from build123d import *

# Parameters (mm, degrees)
BOSS_EXTRUDE5_DEPTH      = 69.85
BOSS_EXTRUDE5_DEPTH_BACK = 19.05
SKETCH1_R                = 25.4
SKETCH1_R_2              = 2.38125
SKETCH1_R_3              = 15.875
SKETCH2_R                = 190.5
SKETCH2_R_2              = 25.4
BOSS_EXTRUDE7_DEPTH      = 69.85
SKETCH4_R                = 190.5
SKETCH4_R_2              = 25.4
CUT_EXTRUDE2_DEPTH       = 19.05
FILLET1_R                = 25.4


with BuildPart() as part:
    # Sketch1 → Boss-Extrude5 (new, two sides: drawn at the far end of the back side and taken through both)
    with BuildSketch(Plane(origin=(0, 0, 0), x_dir=(1, 0, 0), z_dir=(0, 1, 0)).offset(-BOSS_EXTRUDE5_DEPTH_BACK)):
        with Locations(Location((0, 0, 0), (0, 0, 270))):
            Circle(SKETCH1_R)
        with Locations(Location((-8.954275666, 18.593745011, 0), (0, 0, 270))):
            Circle(SKETCH1_R_2, mode=Mode.SUBTRACT)
        with Locations(Location((-16.135047219, 12.867270786, 0), (0, 0, 270))):
            Circle(SKETCH1_R_2, mode=Mode.SUBTRACT)
        with Locations(Location((-20.120074788, 4.592275775, 0), (0, 0, 270))):
            Circle(SKETCH1_R_2, mode=Mode.SUBTRACT)
        with Locations(Location((-20.120074788, -4.592275775, 0), (0, 0, 270))):
            Circle(SKETCH1_R_2, mode=Mode.SUBTRACT)
        with Locations(Location((-16.135047219, -12.867270786, 0), (0, 0, 270))):
            Circle(SKETCH1_R_2, mode=Mode.SUBTRACT)
        with Locations(Location((-8.954275666, -18.593745011, 0), (0, 0, 270))):
            Circle(SKETCH1_R_2, mode=Mode.SUBTRACT)
        with Locations(Location((0, -20.6375, 0), (0, 0, 270))):
            Circle(SKETCH1_R_2, mode=Mode.SUBTRACT)
        with Locations(Location((8.954275666, -18.593745011, 0), (0, 0, 270))):
            Circle(SKETCH1_R_2, mode=Mode.SUBTRACT)
        with Locations(Location((16.135047219, -12.867270786, 0), (0, 0, 270))):
            Circle(SKETCH1_R_2, mode=Mode.SUBTRACT)
        with Locations(Location((20.120074788, -4.592275775, 0), (0, 0, 270))):
            Circle(SKETCH1_R_2, mode=Mode.SUBTRACT)
        with Locations(Location((20.120074788, 4.592275775, 0), (0, 0, 270))):
            Circle(SKETCH1_R_2, mode=Mode.SUBTRACT)
        with Locations(Location((16.135047219, 12.867270786, 0), (0, 0, 270))):
            Circle(SKETCH1_R_2, mode=Mode.SUBTRACT)
        with Locations(Location((8.954275666, 18.593745011, 0), (0, 0, 270))):
            Circle(SKETCH1_R_2, mode=Mode.SUBTRACT)
        with Locations(Location((0, 20.6375, 0), (0, 0, 270))):
            Circle(SKETCH1_R_2, mode=Mode.SUBTRACT)
        with Locations(Location((0, 0, 0), (0, 0, 270))):
            Circle(SKETCH1_R_3, mode=Mode.SUBTRACT)
    extrude(amount=BOSS_EXTRUDE5_DEPTH + BOSS_EXTRUDE5_DEPTH_BACK)

    # Sketch2 → Boss-Extrude7 (add)
    with BuildSketch(Plane(origin=(0, -19.05, 0), x_dir=(-1, 0, 0), z_dir=(0, -1, 0))):
        with Locations(Location((0, 0, 0), (0, 0, 90))):
            Circle(SKETCH2_R)
        with Locations(Location((0, 0, 0), (0, 0, 270))):
            Circle(SKETCH2_R_2, mode=Mode.SUBTRACT)
    extrude(amount=-BOSS_EXTRUDE7_DEPTH)

    # Sketch4 → Cut-Extrude2 (cut)
    with BuildSketch(Plane(origin=(0, -19.05, 0), x_dir=(-1, 0, 0), z_dir=(0, -1, 0))):
        with Locations(Location((0, 0, 0), (0, 0, 90))):
            Circle(SKETCH4_R)
        with Locations(Location((0, 0, 0), (0, 0, 270))):
            Circle(SKETCH4_R_2, mode=Mode.SUBTRACT)
    extrude(amount=-CUT_EXTRUDE2_DEPTH, mode=Mode.SUBTRACT)

    # Fillet1
    fillet1_edges = [part.edges().sort_by_distance(p)[0] for p in [
        (0, 50.8, 190.5),
        (0, 0, 190.5),
    ]]
    fillet(fillet1_edges, radius=FILLET1_R - 0.0001)  # a hair under: the kernel refuses the full size


solid = part.part
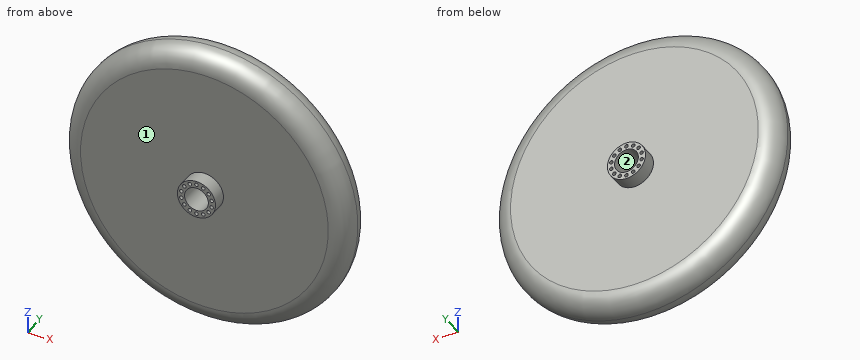
Work out the finished part from the listing and answer in its coordinate system (mm). Face numbers are marked on the shaded views. Give positions to 0.01 mm unless a question says otherwise; leave off trailing zeros. Use a Markdown table: item, result. Add a question column.
1) Consider line 1 along Y through (x, z) = (-100, -13.5); line 2 along X through (y, z) = (65, -5); line 3 along Z through (x, y) = (19, 5.5). Determine where each line is inside the solid, lowest interval first.
2) The part is cut by section A-A, the plane y = -12. Count the separate pieces of the cut face and the enclosed holes in it, plus the area to 3 significant figures.
3) For a pull along X with two mould halves and no side action, classify the marked faces 1 and 2 as +X half, -X half, draft (parallel to the pull), parting line (faces both ways), or undercut.
4) Each of these flat-tipped pins is pushed along its axis until it touches: P1, Ø3, axis at x = 120.5, z = -118, coming from the +Y side; P2, Ø1, axis at x = 8.5, z = -109.5, coming from the -Y side; P3, Ø3, axis at x = -20.12, z = -4.59, coming from the -Y side; P4, Ø1.5, axis at x = -82, y = 14, coming from the -Z side. Where does it stop, or does it pass through?
Reported:
| question | item | result |
|---|---|---|
| 1 | line 1 | y = 0 to 50.8 |
| 1 | line 2 | x = -24.9 to -22.47, -17.77 to -15.07, 15.07 to 17.77, 22.47 to 24.9 |
| 1 | line 3 | z = -179.88 to -6.69, -2.49 to 2.49, 6.69 to 179.88 |
| 2 | separate pieces | 1 |
| 2 | enclosed holes | 15 |
| 2 | area | 986 mm^2 |
| 3 | face 1 | draft |
| 3 | face 2 | undercut |
| 4 | P1 | stops at y = 50.72 |
| 4 | P2 | stops at y = 0 |
| 4 | P3 | passes through |
| 4 | P4 | stops at z = -169.49 |
